Geometry check sheet. Reference: the model listing, model coordinates, mm. Face numbers are marked on the shaded views. A direction names the side the tool comes from. Give positions to 0.01 mm unless a question says otherwise; leave off trailing zeros. Order: outer loops, then holes, each group sorted by start corner. A loop starts at its lowest first (then second) coordinate and runs counter-clockwise, first axis right, second up.
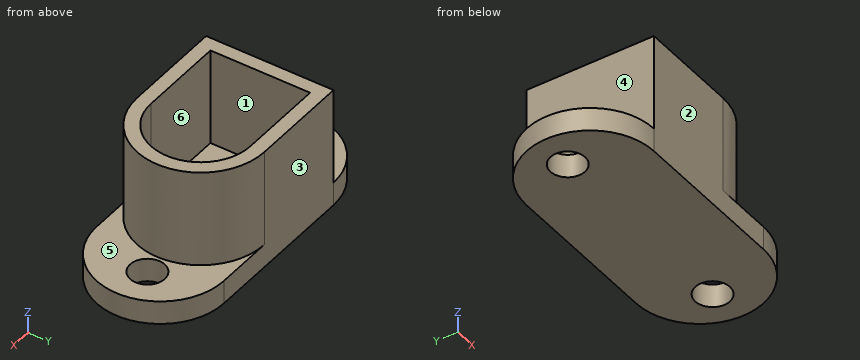
```python
from build123d import *

# Parameters (mm, degrees)
BOSS_EXTRU_1_DEPTH = 7
ESQUISSE2_R        = 1.25
BOSS_EXTRU_2_DEPTH = 1.7


with BuildPart() as part:
    # Esquisse1 → Boss.-Extru.1 (new body)
    with BuildSketch(Plane.XY):
        with BuildLine():
            Line((-7.25, -4.6), (-7.25, 4.6))
            Line((-7.25, 4.6), (0, 4.6))
            ThreePointArc((0, 4.6), (4.6, 0), (0, -4.6))
            Line((0, -4.6), (-7.25, -4.6))
        make_face()
        with BuildLine():
            Line((-6.25, -3.6), (-6.25, 3.6))
            Line((-6.25, 3.6), (0, 3.6))
            ThreePointArc((0, 3.6), (3.6, 0), (0, -3.6))
            Line((0, -3.6), (-6.25, -3.6))
        make_face(mode=Mode.SUBTRACT)
    extrude(amount=BOSS_EXTRU_1_DEPTH)

    # Esquisse2 → Boss.-Extru.2 (add)
    with BuildSketch(Plane(origin=(0, 0, 0), x_dir=(-1, 0, 0), z_dir=(0, 0, -1))):
        with BuildLine():
            Line((7.25, 4.6), (-4.25, 4.6))
            ThreePointArc((-4.25, 4.6), (-8.85, 0), (-4.25, -4.6))
            Line((-4.25, -4.6), (7.25, -4.6))
            ThreePointArc((7.25, -4.6), (11.85, 0), (7.25, 4.6))
        make_face()
        with Locations((9.1, 0.35)):
            Circle(ESQUISSE2_R, mode=Mode.SUBTRACT)
        with Locations((-6.1, 0.35)):
            Circle(ESQUISSE2_R, mode=Mode.SUBTRACT)
    extrude(amount=BOSS_EXTRU_2_DEPTH)


solid = part.part
```
Q1. Gauge pin test, flat ends, axial feed: P1, Ø2, axis at x = 1, z = 6, coming from the +Y side; P2, Ø2, axis at y = 1.5, z = 4, coming from the +X side; P3, Ø2.5, axis at x = -10.5, y = 0.5, coming from the +Z side; P4, Ø2, axis at y = -1.5, z = 6, coming from the -X side. Record the tip position at first contact, or that the pin passes through.
Q2. Thickness scan on L1, parallel to Y at x = -4.25, z = 1.75; L2, parallel to Z at x = 6, y = 3; L3, parallel to X at y = 0, z = -1. Record the ranges inside material, lowest first.
Q3. Cross-section at B-B, the plane y = 0.35. Record the boundary of the cut face in (x, z), and give its area (3 significant figures).
Q4. Cross-section at C-C, the plane x = -9.1. Record the boundary of the cut face in (y, z).
Q5. Cross-section at D-D, the plane x = -1. Record the boundary of the cut face in (y, z).
Q6. Cross-section at A-A, the plane z = 2.5. Record the boundary of the cut face in (x, y), and give its area (3 significant figures).
Q7. Release check for a two-part mould opening along Y. For the marked faces 1, 2 and 3 record: pulls with the +Y half, pulls with the -Y half, needs draft (parallel to the pull), parting line crosses it, or undercut.
Q8. Access from +Z, -Z, +X, -X, +Y, -Y to the whole of each face (thin tool, end or side, straight path). Record for the marked faces 4, 5 and 6.
Answers follow:
1. P1: stops at y = 4.6
1. P2: stops at x = 4.57
1. P3: stops at z = 0
1. P4: stops at x = -7.25
2. L1: y = -4.6 to -3.6, 3.6 to 4.6
2. L2: z = -1.7 to 0
2. L3: x = -11.85 to -10.3, -7.9 to 4.9, 7.3 to 8.85
3. outline: (-11.84, -1.7) - (-10.35, -1.7) - (-10.35, 0) - (-11.84, 0) - close; (-7.85, -1.7) - (4.85, -1.7) - (4.85, 0) - (4.59, 0) - (4.59, 7) - (3.58, 7) - (3.58, 0) - (-6.25, 0) - (-6.25, 7) - (-7.25, 7) - (-7.25, 0) - (-7.85, 0) - close; (7.35, -1.7) - (8.84, -1.7) - (8.84, 0) - (7.35, 0) - close
3. area: 40.7 mm2
4. outline: (-4.21, -1.7) - (-0.9, -1.7) - (-0.9, 0) - (-4.21, 0) - close; (1.6, -1.7) - (4.21, -1.7) - (4.21, 0) - (1.6, 0) - close
5. outline: (-4.6, -1.7) - (4.6, -1.7) - (4.6, 7) - (3.6, 7) - (3.6, 0) - (-3.6, 0) - (-3.6, 7) - (-4.6, 7) - close
6. outline: (-7.25, -4.6) - (0, -4.6) arc R4.6 ccw to (0, 4.6) - (-7.25, 4.6) - close; hole (-6.25, -3.6) - (0, -3.6) arc R3.6 ccw to (0, 3.6) - (-6.25, 3.6) - close
6. area: 34.6 mm2
7. face 1: undercut
7. face 2: pulls with the -Y half
7. face 3: pulls with the +Y half
8. face 4: +Z, -X, +Y, -Y
8. face 5: +Z, +X
8. face 6: +Z
